Autodesk Fusion 360 part; units mm, degrees
sketch "Sketch1" plane through (0, 0, 0) normal (0, 0, 1) x (1, 0, 0)
  line L0 (0, 0) -> (89.0778, 0)
  line L1 (89.0778, 0) -> (89.0778, 41.3004)
  line L2 (89.0778, 41.3004) -> (0, 41.3004)
  line L3 (0, 41.3004) -> (0, 0)
  line L4 (0, 41.3004) -> (6.35, 41.3004)
  line L5 (6.35, 41.3004) -> (6.35, 0)
  line L6 (6.35, 0) -> (0, 0)
  line L7 (0, 0) -> (0, 41.3004)
  circle A0 centre (33.4171, 20.6502) radius 9.525
  circle A1 centre (68.046, 20.6502) radius 9.525
  point P0 (50.7316, 20.6502)
  dimension "d1" = 89.0778
  dimension "d2" = 41.3004
  dimension "d7" = 6.35
  dimension "d12" = 19.05
  dimension "d19" = 17.3145
  dimension "d20" = 17.3145
extrude "Extrude1" add sketch "Sketch1" along normal blind 6.35 contours L0 L2 L3 L4 L5 L6 L7 | L0 L1 L2 L5 | A0 | A1
extrude "Extrude2" add sketch "Sketch1" along normal blind 104.648 contours L0 L2 L3 L4 L5 L6 L7
fillet "Fillet1" radius 6.35 1 edges at (0, 20.6502, 0)
extrude "Extrude3" cut sketch "Sketch1" along normal blind 129.54 contours A0 | A1
sketch "Sketch2" plane through (0, 0, 0) normal (-1, 0, 0) x (0, -1, 0)
  line L0 (-41.3004, 6.35) -> (0, 6.35)
  line L1 (0, 6.35) -> (0, 104.648)
  line L2 (0, 104.648) -> (-41.3004, 104.648)
  line L3 (-41.3004, 104.648) -> (-41.3004, 6.35)
  line L4 (-20.6502, 104.648) -> (-20.6502, 6.35) construction
  circle A0 centre (-20.6502, 72.4894) radius 9.525
  circle A1 centre (-20.6502, 35.7876) radius 9.525
  dimension "d15" = 19.05
  dimension "d16" = 19.05
extrude "Extrude4" cut sketch "Sketch2" against normal blind 182.88 contours A0 | A1
equation "d20 = d19"
The model under review builds one solid part; all positions refer to its coordinate system, in mm. A direction names the side the tool comes from. Round coordinates to 2 decimals unless told otherwise and drop trailing zeros. Order: outer loops, then holes, each group sorted by start corner. A loop starts at its lowest first (then second) coordinate and runs counter-clockwise, first axis right, second up.
(1) Take a section at D-D, the plane y = 5.5. State the section outline as (x, z) points.
Working result:
outline: (0, 6.35) arc R6.35 ccw to (6.35, 0) - (89.08, 0) - (89.08, 6.35) - (6.35, 6.35) - (6.35, 104.65) - (0, 104.65) - close
(2) Take a section at A-A, the plane x = 75.5. State the section outline as (y, z) points, plus the area to 3 significant figures.
Working result:
outline: (0, 0) - (14.72, 0) - (14.72, 6.35) - (0, 6.35) - close; (26.58, 0) - (41.3, 0) - (41.3, 6.35) - (26.58, 6.35) - close
area: 187 mm2
(3) Take a section at C-C, the plane z = 78.5. State the section outline as (x, y) points, plus the area to 3 significant figures.
Working result:
outline: (0, 0) - (6.35, 0) - (6.35, 13.26) - (0, 13.26) - close; (0, 28.04) - (6.35, 28.04) - (6.35, 41.3) - (0, 41.3) - close
area: 168 mm2
(4) Take a section at B-B, the plane y = 24. State the section outline as (x, z) points, plus the area to 3 significant figures.
Working result:
outline: (0, 6.35) arc R6.35 ccw to (6.35, 0) - (24.5, 0) - (24.5, 6.35) - (6.35, 6.35) - (6.35, 26.87) - (0, 26.87) - close; (0, 44.7) - (6.35, 44.7) - (6.35, 63.57) - (0, 63.57) - close; (0, 81.41) - (6.35, 81.41) - (6.35, 104.65) - (0, 104.65) - close; (42.33, 0) - (59.13, 0) - (59.13, 6.35) - (42.33, 6.35) - close; (76.96, 0) - (89.08, 0) - (89.08, 6.35) - (76.96, 6.35) - close
area: 728 mm2
(5) For P1, Ø5, axis at x = 16, y = 30, coming from the +Z side; P2, Ø5, axis at y = 11, z = 44, coming from the +X side, all flat-tipped, find the tip position at first contact; note any pin that passes through.
Working result:
P1: stops at z = 6.35
P2: stops at x = 6.35
(6) Wall thickness on L1, parallel to Z at x = 49, y = 18.5: over which ranges is the line inside the solid? List them lowest first.
Working result:
L1: z = 0 to 6.35
(7) Tool access review of faces 1 (the face through (1.81, 20.36, 1.91)), 2 (the face through (6.35, 21, 55)): name each direction out of +Z, -Z, +X, -X, +Y, -Y from which nothing blocks a thin tool from reaching the whole face with its end or side.
Working result:
face 1: -Z, -X, +Y, -Y
face 2: +Z, +X, +Y, -Y
(8) Mouldability with a two-part tool opening along Y and no side actions: class faces 3 (the face through (5, 41.3, 29)), 4 (the face through (89.078, 20, 3)), 5 (the face through (31.35, 29.95, 3.13)) as released by +Y, released by -Y, zero draft, split by the parting line, or undercut.
Working result:
face 3: released by +Y
face 4: zero draft
face 5: undercut
